The listing builds one solid part. Answer for the finished solid, in the listing's coordinates (mm). Coordinates: 2 decimals unless noted, no trailing zeros. Loops run counter-clockwise (first coordinate to the right, second up) from the corner with the lowest first, then second, coordinate; pieces in that order, holes last. Notation, with made-up numbers: M -36.5,33 L 5.5,33 A27 ccw 5.5,62 Z; hole C 40.5,62.25 d8. An arc over 180 degrees is marked long. Return JSON: item names as keys, results as strings. Group by question number.
1. Section D-D (y = 5.5) is taken. Write down the section's boundary in (x, z), then the cut area to 3 significant figures.
2. Section A-A (y = 21.5) is taken. Write down the section's boundary in (x, z), then the cut area to 3 significant figures.
3. Section B-B (z = 1.5) is taken. Write down the section's boundary in (x, y).
4. Section C-C (x = 9) is taken. Write down the section's boundary in (y, z).
5. Given P1, Ø1, axis at y = 37.5, z = 1.5, coming from the -X side; P2, Ø3, axis at x = 6, y = 10, coming from the -Z side; P3, Ø0.6, axis at y = 42.5, z = 0.5, coming from the +X side; P4, Ø0.6, axis at x = 19, z = 1, coming from the +Y side, each flat-ended and moving along its own axis, determine where each tip first touches the part or whether it passes through.
6. Straight lines are drawn through the part: L1, parallel to Y at x = 9, z = 1.4; L2, parallel to Y at x = 10, z = 1.35; L3, parallel to X at y = 16, z = 0.55. For each, find the intervals that lie inside material, in ascending order. Write a range as from..to.
```python
from build123d import *

# Parameters (mm, degrees)
EXTRUDE_1_DEPTH     = 2
SKETCH_2_R          = 1.6
CUT_EXTRUDE_1_DEPTH = 3
SKETCH_3_W          = 3
SKETCH_3_H          = 24
SKETCH_3_W_2        = 4
CUT_EXTRUDE_2_DEPTH = 3
SKETCH_4_W          = 10
SKETCH_4_H          = 2
EXTRUDE_2_DEPTH     = 2
SKETCH_5_R          = 0.75
CUT_EXTRUDE_3_DEPTH = 3


with BuildPart() as part:
    # 草图1 → 凸台-拉伸1 (new body)
    with BuildSketch(Plane.XY):
        Polygon((0, 0), (17, 0), (17, 2.5), (20, 2.5), (20, 14.5), (17, 14.5), (17, 51.5), (0, 51.5), align=None)
    extrude(amount=EXTRUDE_1_DEPTH)

    # 草图2 → 切除-拉伸1 (cut, through all)
    with BuildSketch(Plane.XY.offset(2)):
        with Locations((9, 5.5)):
            Circle(SKETCH_2_R)
        with Locations((9, 21.5)):
            Circle(SKETCH_2_R)
    extrude(amount=-CUT_EXTRUDE_1_DEPTH, mode=Mode.SUBTRACT)

    # 草图3 → 切除-拉伸2 (cut, through all)
    with BuildSketch(Plane.XY.offset(2)):
        with Locations((15.5, 39.5)):
            Rectangle(SKETCH_3_W, SKETCH_3_H)
        with Locations((2, 39.5)):
            Rectangle(SKETCH_3_W_2, SKETCH_3_H)
    extrude(amount=-CUT_EXTRUDE_2_DEPTH, mode=Mode.SUBTRACT)

    # 草图4 → 凸台-拉伸2 (add)
    with BuildSketch(Plane(origin=(0, 51.5, 0), x_dir=(1, 0, 0), z_dir=(0, 1, 0))):
        with Locations((9, -1)):
            Rectangle(SKETCH_4_W, SKETCH_4_H)
    extrude(amount=EXTRUDE_2_DEPTH)

    # 草图5 → 切除-拉伸3 (cut)
    with BuildSketch(Plane.XY.offset(2)):
        with Locations((17, 14.5)):
            Circle(SKETCH_5_R)
        with Locations((17, 2.5)):
            Circle(SKETCH_5_R)
    extrude(amount=-CUT_EXTRUDE_3_DEPTH, mode=Mode.SUBTRACT)


solid = part.part
```
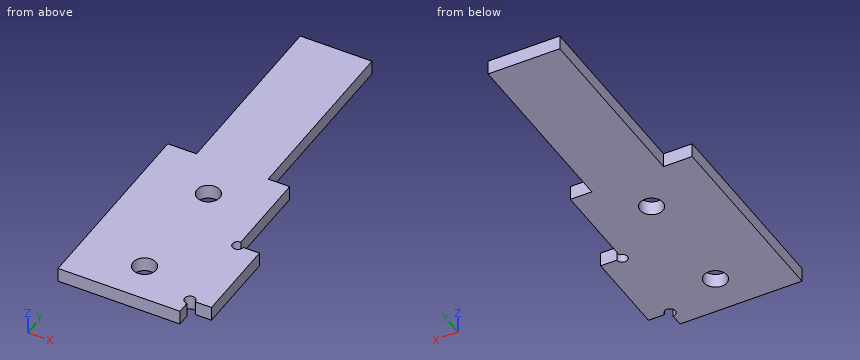
Worked out:
{
 "1": {"outline": "M 0,0 L 7.4,0 L 7.4,2 L 0,2 Z; M 10.6,0 L 20,0 L 20,2 L 10.6,2 Z", "area": "33.6 mm^2"},
 "2": {"outline": "M 0,0 L 7.4,0 L 7.4,2 L 0,2 Z; M 10.6,0 L 17,0 L 17,2 L 10.6,2 Z", "area": "27.6 mm^2"},
 "3": {"outline": "M 0,0 L 17,0 L 17,1.75 A0.75 cw long 17.75,2.5 L 20,2.5 L 20,14.5 L 17.75,14.5 A0.75 cw long 17,15.25 L 17,27.5 L 14,27.5 L 14,53.5 L 4,53.5 L 4,27.5 L 0,27.5 Z; hole C 9,5.5 d3.2; hole C 9,21.5 d3.2"},
 "4": {"outline": "M 0,0 L 3.9,0 L 3.9,2 L 0,2 Z; M 7.1,0 L 19.9,0 L 19.9,2 L 7.1,2 Z; M 23.1,0 L 53.5,0 L 53.5,2 L 23.1,2 Z"},
 "5": {"P1": "x = 4", "P2": "z = 0", "P3": "x = 14", "P4": "y = 14.5"},
 "6": {"L1": "0..3.9, 7.1..19.9, 23.1..53.5", "L2": "0..4.25, 6.75..20.25, 22.75..53.5", "L3": "0..17"}
}
